from build123d import *

# Parameters (mm, degrees)
ESTRUSIONE_ESTRUSIONE1_DEPTH = 2
SCHIZZO2_R                   = 1.5
TAGLIO_ESTRUSIONE1_DEPTH     = 59.798875742


with BuildPart() as part:
    # Schizzo1 → Estrusione-Estrusione1 (new body)
    with BuildSketch(Plane.XY):
        Polygon((0, 55.815504809), (2.15, 57.907752405), (7.85, 57.907752405), (10, 55.815504809), (10, 0), (7.85, -2.092247595), (2.15, -2.092247595), (0, 0), align=None)
    extrude(amount=-ESTRUSIONE_ESTRUSIONE1_DEPTH)

    # Schizzo2 → Taglio-Estrusione1 (cut, through all)
    with BuildSketch(Plane.XY):
        with Locations((5, 51.907752405)):
            Circle(SCHIZZO2_R)
        with Locations((5, 3.907752405)):
            Circle(SCHIZZO2_R)
    extrude(amount=-TAGLIO_ESTRUSIONE1_DEPTH, mode=Mode.SUBTRACT)


solid = part.part
Source: CAD feature listing. Evaluate the final solid. Frame: model axes, mm. Give positions to 0.01 mm unless a question says otherwise; leave off trailing zeros. Write each loop counter-clockwise with the first axis right and the second up, starting at its lowest first coordinate (ties: lowest second). Pieces come first, ordered by that corner, then holes. Notation, with made-up numbers: M 15.25,-34 L 48.25,-34 A16 cw 48.25,-27 Z; hole C 29.25,25 d3. An arc over 180 degrees is marked long. Return JSON: item names as keys, results as strings. Group by question number.
1) Cut plane C-C, the plane x = 1. Output: boundary loops of the cut face in (y, z).
2) Cut plane D-D, the plane x = 9.5. Output: boundary loops of the cut face in (y, z), plus the area to 3 significant figures.
3) Cut plane A-A, the plane x = 5. Output: boundary loops of the cut face in (y, z), plus the area to 3 significant figures.
4) Pull-direction query (Y, two-part tool) for faces 1 (the face through (1.06, 56.847, -0.986)), 2 (the face through (10, 28, -1)), 3 (the face through (5.81, 5.17, -0.99)); classes: pulls with the +Y half, pulls with the -Y half, needs draft (parallel to the pull), parting line crosses it, or undercut.
5) Cut plane B-B, the plane z = -1.05. Output: boundary loops of the cut face in (x, y), plus the area to 3 significant figures.
6) Material intervals for line 1 along Y through (x, z) = (5, -1.35); line 2 along X through (y, z) = (3, -0.5); line 3 along Y through (x, z) = (8, -1.35), sorted ascending. Write a range as [from, to].
Recorded:
{
 "1": {"outline": "M -0.97,-2 L 56.79,-2 L 56.79,0 L -0.97,0 Z"},
 "2": {"outline": "M -0.49,-2 L 56.3,-2 L 56.3,0 L -0.49,0 Z", "area": "114 mm²"},
 "3": {"outline": "M -2.09,-2 L 2.41,-2 L 2.41,0 L -2.09,0 Z; M 5.41,-2 L 50.41,-2 L 50.41,0 L 5.41,0 Z; M 53.41,-2 L 57.91,-2 L 57.91,0 L 53.41,0 Z", "area": "108 mm²"},
 "4": {"face 1": "pulls with the +Y half", "face 2": "needs draft", "face 3": "undercut"},
 "5": {"outline": "M 0,0 L 2.15,-2.09 L 7.85,-2.09 L 10,0 L 10,55.82 L 7.85,57.91 L 2.15,57.91 L 0,55.82 Z; hole C 5,3.91 d3; hole C 5,51.91 d3", "area": "577 mm²"},
 "6": {"line 1": "y = [-2.09, 2.41], [5.41, 50.41], [53.41, 57.91]", "line 2": "x = [0, 3.81], [6.19, 10]", "line 3": "y = [-1.95, 57.76]"}
}
